Here's how the part is built. I have some questions about the finished solid (model axes, mm). Face numbers are marked on the shaded views. A direction names the side the tool comes from. Give positions to 0.01 mm unless a question says otherwise; leave off trailing zeros. Loops run counter-clockwise (first coordinate to the right, second up) from the corner with the lowest first, then second, coordinate; pieces in that order, holes last.
Q1. If we section it at C-C (y = 2.5): Please give me the cut outline in (x, z), plus the area to 3 significant figures.
Q2. I need wall thicknesses on line 1 (X direction, y = 7.75, z = 0); line 2 (Z direction, x = -4.5, y = 6); line 3 (X direction, y = 6.25, z = 11.5). Which ranges of each line are inside material? Lowest first, please.
Q3. Will these pins go through, and if not, where does the flat tip stop? P1, Ø3, axis at x = -7.5, y = 8.5, coming from the -Z side; P2, Ø7, axis at x = 21.41, z = 8.82, coming from the -Y side; P3, Ø2, axis at x = -14.5, y = 3.5, coming from the +Z side.
Q4. If we section it at A-A (x = 0): Please give me the cut outline in (y, z).
Q5. We'd pull the mould along X, two halves only. Please class the marked faces 1, 2 and 3: +X half, -X half, draft (parallel to the pull), parting line (faces both ways), or undercut.
Q6. For the marked faces 4 and 5, which set-ups out of +Z, -Z, +X, -X, +Y, -Y let a thin tool reach every point of the face, with its end or its side?
Q7. If we section it at B-B (z = 0): Please give me the cut outline in (x, y).
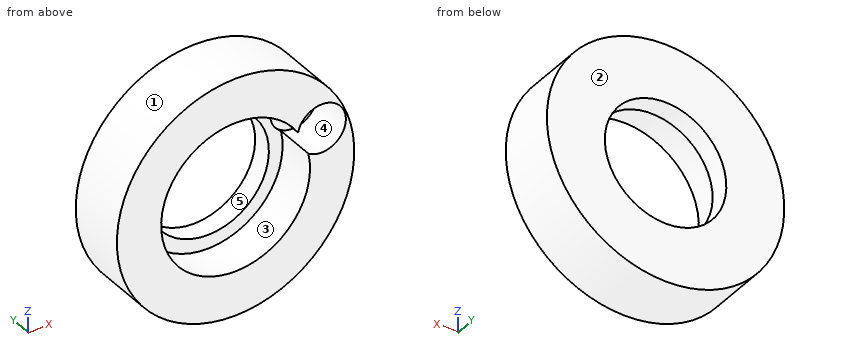
from build123d import *

# Parameters (mm, degrees)
SKETCH1_R           = 29.5
BOSS_EXTRUDE1_DEPTH = 15
SKETCH2_R           = 15.1
CUT_EXTRUDE1_DEPTH  = 45.333959895
SKETCH3_R           = 18.5
CUT_EXTRUDE2_DEPTH  = 10
SKETCH4_R           = 6
CUT_EXTRUDE3_DEPTH  = 10.5


with BuildPart() as part:
    # Sketch1 → Boss-Extrude1 (new body)
    with BuildSketch(Plane(origin=(0, 0, 0), x_dir=(1, 0, 0), z_dir=(0, 1, 0))):
        with Locations(Location((0, 0, 0), (0, 0, 270))):
            Circle(SKETCH1_R)
    extrude(amount=BOSS_EXTRUDE1_DEPTH)

    # Sketch2 → Cut-Extrude1 (cut, through all)
    with BuildSketch(Plane.XZ):
        with Locations(Location((0, 0, 0), (0, 0, 270))):
            Circle(SKETCH2_R)
    extrude(amount=-CUT_EXTRUDE1_DEPTH, mode=Mode.SUBTRACT)

    # Sketch3 → Cut-Extrude2 (cut)
    with BuildSketch(Plane.XZ):
        with Locations(Location((0, 0, 0), (0, 0, 270))):
            Circle(SKETCH3_R)
    extrude(amount=-CUT_EXTRUDE2_DEPTH, mode=Mode.SUBTRACT)

    # Sketch4 → Cut-Extrude3 (cut)
    with BuildSketch(Plane.XZ):
        with Locations(Location((21.406403657, 8.819380288, 0), (0, 0, 270))):
            Circle(SKETCH4_R)
    extrude(amount=-CUT_EXTRUDE3_DEPTH, mode=Mode.SUBTRACT)


solid = part.part
Check sheet entries:
1. outline: circle Ø59 at (0, 0); hole (15.53, 10.05) arc R18.5 ccw (long way) to (18.1, 3.81) arc R6 ccw (long way) to start
1. area: 1,550 mm2
2. line 1: x = -29.5 to -18.5, 18.5 to 29.5
2. line 2: z = -29.15 to -17.94, 17.94 to 29.15
2. line 3: x = -27.17 to -14.49, 14.49 to 16.04, 26.77 to 27.17
3. P1: stops at z = -28.88
3. P2: stops at y = 10.5
3. P3: stops at z = 26.23
4. outline: (0, -29.5) - (15, -29.5) - (15, -15.1) - (10, -15.1) - (10, -18.5) - (0, -18.5) - close; (0, 18.5) - (10, 18.5) - (10, 15.1) - (15, 15.1) - (15, 29.5) - (0, 29.5) - close
5. face 1: parting line
5. face 2: draft
5. face 3: undercut
6. face 4: -Y
6. face 5: +Y, -Y
7. outline: (-29.5, 0) - (-18.5, 0) - (-18.5, 10) - (-15.1, 10) - (-15.1, 15) - (-29.5, 15) - close; (15.1, 10) - (18.5, 10) - (18.5, 0) - (29.5, 0) - (29.5, 15) - (15.1, 15) - close
